Here's how the part is built. I have some questions about the finished solid (model axes, mm). A direction names the side the tool comes from. Round coordinates to 2 decimals unless told otherwise and drop trailing zeros. Write each loop counter-clockwise with the first axis right and the second up, starting at its lowest first coordinate (ties: lowest second). Pieces come first, ordered by that corner, then holes. Notation, with made-up numbers: (-8.75, 52.5) - (28.25, 52.5) arc R16 ccw to (28.25, 74.5) - close; hole circle Ø2 at (26.25, -39). An arc over 180 degrees is marked (long way). Write item = value, one per line. Start each with the question number.
Item 1: If we section it at C-C (y = -20.5): Please give me the cut outline in (x, z).
Item 2: If we section it at D-D (x = 13.75): Please give me the cut outline in (y, z).
Item 3: If we section it at B-B (x = -16): Please give me the cut outline in (y, z).
Item 4: If we section it at A-A (y = 0): Please give me the cut outline in (x, z).
Item 5: For P1, Ø3, axis at x = 13.75, y = -23.82, coming from the +Z side; P2, Ø1, axis at x = -25.5, z = 1.5, coming from the +Y side, each with a flat end and sliding along its axis, tell me the tip position at first contact or that it passes through.
Item 6: If I drill on line 1 along Y through (x, z) = (13.75, 0.9); line 2 along X through (y, z) = (8.5, 1.7); line 3 along X through (y, z) = (27.5, 1.8), over which ranges is the centre line in solid material (lowest first)? Write a range as [from, to].
Item 7: Which directions (+Z, -Z, +X, -X, +Y, -Y) give clear straight access to the entire face, cutting with the end or side of a thin tool? Please do faces 1 (the face through (8, -25, 2)), 2 (the face through (-15.17, -25.88, 0.99)).
Item 8: Thinking about a two-plate mould opening in X: for faces 3 (the face through (8, -25, 0)), 4 (the face through (-5.077, 38.668, 0.986)), 5 (the face through (-14.83, 26.08, 0.99)), which applies, pulls with the +X half, pulls with the -X half, needs draft (parallel to the pull), parting line crosses it, or undercut?
```python
from build123d import *

# Parameters (mm, degrees)
SKETCH_1_R        = 39
EXTRUDE_1_DEPTH   = 2
FILLET_1_R        = 10
HOLE_WIZARD_M31_D = 3.4


with BuildPart() as part:
    # Эскиз1 → Бобышка-Вытянуть1 (new body)
    with BuildSketch(Plane.XY):
        Circle(SKETCH_1_R)
        with BuildLine():
            ThreePointArc((20.612446655, -21.797409087), (30, 0), (20.612446655, 21.797409087))
            ThreePointArc((20.612446655, 21.797409087), (11.5, 19.918584287), (8.570886678, 28.749606981))
            ThreePointArc((8.570886678, 28.749606981), (-15, 25.980762114), (-29.183333333, 6.952197894))
            ThreePointArc((-29.183333333, 6.952197894), (-23, 0), (-29.183333333, -6.952197894))
            ThreePointArc((-29.183333333, -6.952197894), (-15, -25.980762114), (8.570886678, -28.749606981))
            ThreePointArc((8.570886678, -28.749606981), (11.5, -19.918584287), (20.612446655, -21.797409087))
        make_face(mode=Mode.SUBTRACT)
    extrude(amount=EXTRUDE_1_DEPTH)

    # Скругление1
    fillet_1_edges = [part.edges().sort_by_distance(p)[0] for p in [
        (-29.183333333, 6.952197894, 1),
        (-29.183333333, -6.952197894, 1),
        (8.570886678, -28.749606981, 1),
        (20.612446655, -21.797409087, 1),
        (20.612446655, 21.797409087, 1),
        (8.570886678, 28.749606981, 1),
    ]]
    fillet(fillet_1_edges, radius=FILLET_1_R)

    # Отверстие с зазором M31 (through all)
    with Locations(Plane.XY.offset(2)):
        with Locations((13.75, 23.815698604), (-27.5, 0), (13.75, -23.815698604)):
            Hole(HOLE_WIZARD_M31_D / 2)


solid = part.part
```
Reply:
q1.outline = (-33.18, 0) - (-21.9, 0) - (-21.9, 2) - (-33.18, 2) - close; (10.65, 0) - (33.18, 0) - (33.18, 2) - (10.65, 2) - close
q2.outline = (-36.5, 0) - (-25.52, 0) - (-25.52, 2) - (-36.5, 2) - close; (-22.12, 0) - (-19.09, 0) - (-19.09, 2) - (-22.12, 2) - close; (19.09, 0) - (22.12, 0) - (22.12, 2) - (19.09, 2) - close; (25.52, 0) - (36.5, 0) - (36.5, 2) - (25.52, 2) - close
q3.outline = (-35.57, 0) - (-25.38, 0) - (-25.38, 2) - (-35.57, 2) - close; (25.38, 0) - (35.57, 0) - (35.57, 2) - (25.38, 2) - close
q4.outline = (-39, 0) - (-29.2, 0) - (-29.2, 2) - (-39, 2) - close; (-25.8, 0) - (-23, 0) - (-23, 2) - (-25.8, 2) - close; (30, 0) - (39, 0) - (39, 2) - (30, 2) - close
q5.P1 = through
q5.P2 = 29.93
q6.line_1 = [-36.5, -25.52], [-22.12, -19.09], [19.09, 22.12], [25.52, 36.5]
q6.line_2 = [-38.06, -26.59], [28.77, 38.06]
q6.line_3 = [-27.65, -11.99], [5.69, 27.65]
q7.face_1 = +Z, +X, -X, +Y, -Y
q7.face_2 = +Z, -Z
q8.face_3 = needs draft
q8.face_4 = parting line crosses it
q8.face_5 = undercut
